Check sheet for the modelled part. Datum: model origin and axes. Units: mm. Round coordinates to 2 decimals unless told otherwise and drop trailing zeros. Write each loop counter-clockwise with the first axis right and the second up, starting at its lowest first coordinate (ties: lowest second). Pieces come first, ordered by that corner, then holes.
Item 1: Cross-section at C-C on z = 7.5. Enter the section's corners in (x, y), plus the area to 3 significant figures.
Item 2: Cross-section at D-D on y = 45.5. Enter the section's corners in (x, z).
Item 3: Material ranges on line 1 (Y direction, x = 3, z = 0); line 2 (Z direction, x = 2.5, y = 50); line 3 (Y direction, x = 3.5, z = -3.5), recorded low to high.
Item 4: Go/stop test with flat-tipped pins: pin 1 Ø1 at (x, z) = (2.5, 4.5) entering from +Y; pin 2 Ø1 at (y, z) = (28, -7.5) entering from -X; pin 3 Ø2 at (x, z) = (2.5, -7.5) entering from -Y; pin 4 Ø1 at (x, y) = (2.5, 24) entering from -Z. Record where each tip stops, or that it passes through.
Item 5: Cross-section at B-B on x = 6. Enter the section's corners in (y, z), plus the area to 3 significant figures.
Item 6: Cross-section at A-A on z = 0. Enter the section's corners in (x, y), plus the area to 4 significant figures.
Item 7: Release check for a two-part mould opening along Y. For faces 1 (the cylindrical face through (3.451, 47.273, 0.358)), 2 (the cylindrical face through (3, -10, 0)), 3 (the flat face through (7, 23, 0)) record: +Y half, -Y half, draft (parallel to the pull), parting line (faces both ways), or undercut.
from build123d import *

# Parameters (mm, degrees)
SKETCH1_R             = 5
BOSS_EXTRUDE1_DEPTH   = 7
M10_CLEARANCE_HOLE1_D = 11
M5_CLEARANCE_HOLE1_D  = 5.5


with BuildPart() as part:
    # Sketch1 → Boss-Extrude1 (new body)
    with BuildSketch(Plane(origin=(0, 0, 0), x_dir=(0, 0, -1), z_dir=(1, 0, 0))):
        with Locations((0, 50)):
            Circle(SKETCH1_R)
        with BuildLine():
            ThreePointArc((-4.99342402, 49.743647589), (-5.733969822, 26.838261478), (-9.089996824, 4.167968058))
            ThreePointArc((-9.089996824, 4.167968058), (0, 10), (9.089996824, 4.167968058))
            ThreePointArc((9.089996824, 4.167968058), (5.733969822, 26.838261478), (4.99342402, 49.743647589))
            ThreePointArc((4.99342402, 49.743647589), (0, 45), (-4.99342402, 49.743647589))
        make_face()
        with BuildLine():
            ThreePointArc((-9.089996824, 4.167968058), (-9.533884852, 2.081557577), (-10, 0))
            ThreePointArc((-10, 0), (0, -10), (10, 0))
            ThreePointArc((10, 0), (9.533884852, 2.081557577), (9.089996824, 4.167968058))
            ThreePointArc((9.089996824, 4.167968058), (0, 10), (-9.089996824, 4.167968058))
        make_face()
    extrude(amount=BOSS_EXTRUDE1_DEPTH)

    # M10 Clearance Hole1 (through all)
    with Locations(Plane(origin=(7, 0, 0), x_dir=(0, 0, 1), z_dir=(1, 0, 0))):
        with Locations((0, 0)):
            Hole(M10_CLEARANCE_HOLE1_D / 2)

    # M5 Clearance Hole1 (through all)
    with Locations(Plane(origin=(7, 50, 0), x_dir=(0, 0, 1), z_dir=(1, 0, 0))):
        with Locations((0, 0)):
            Hole(M5_CLEARANCE_HOLE1_D / 2)


solid = part.part
Response values:
1. outline: (0, -6.61) - (7, -6.61) - (7, 12.79) - (0, 12.79) - close
1. area: 136 mm2
2. outline: (0, -4.93) - (7, -4.93) - (7, 4.93) - (0, 4.93) - close
3. line 1: y = -10 to -5.5, 5.5 to 47.25, 52.75 to 55
3. line 2: z = -5 to -2.75, 2.75 to 5
3. line 3: y = -9.37 to -4.24, 4.24 to 53.57
4. pin 1: stops at y = 53
4. pin 2: passes through
4. pin 3: stops at y = -7.6
4. pin 4: stops at z = -6.06
5. outline: (0, -10) arc R200 cw to (4.17, -9.09) arc R200 cw to (49.74, -4.99) arc R5 ccw (long way) to (49.74, 4.99) arc R200 cw to (4.17, 9.09) arc R200 cw to (0, 10) arc R10 ccw to start; hole circle Ø11 at (0, 0); hole circle Ø5.5 at (50, 0)
5. area: 721 mm2
6. outline: (0, -10) - (7, -10) - (7, -5.5) - (0, -5.5) - close; (0, 5.5) - (7, 5.5) - (7, 47.25) - (0, 47.25) - close; (0, 52.75) - (7, 52.75) - (7, 55) - (0, 55) - close
6. area: 339.5 mm2
7. face 1: undercut
7. face 2: -Y half
7. face 3: draft
